Autodesk Inventor part; units mm, degrees
ref_plane "YZ Plane" through (0, 0, 0) normal (1, 0, 0) x (0, 1, 0)
ref_plane "XZ Plane" through (0, 0, 0) normal (0, 1, 0) x (-1, 0, 0)
ref_plane "XY Plane" through (0, 0, 0) normal (0, 0, 1) x (1, 0, 0)
sketch "Sketch1" plane through (0, 0, 0) normal (1, 0, 0) x (0, 1, 0)
  circle A0 centre (0, 0) radius 26.5
  dimension "d0" = 53
extrude "Extrusion1" add sketch "Sketch1" along normal blind 51
sketch "Sketch2" plane through (0, 0, 0) normal (0, 1, 0) x (-1, 0, 0)
  line L0 (-51, 26.5) -> (-51, -26.5)
  circle A0 centre (-51, 0) radius 46
  point P0 (0, 0)
  dimension "d3" = 92
extrude "Extrusion2" add sketch "Sketch2" along normal mid plane 60
move or copy body "Move Body1" bodies to move or copy 1 copy no translate (15, 0, 0)
properties part number "hip"
Model file for the job. Use its own axes, mm. A direction names the side the tool comes from. Give positions to 0.01 mm unless a question says otherwise; leave off trailing zeros. Loops run counter-clockwise (first coordinate to the right, second up) from the corner with the lowest first, then second, coordinate; pieces in that order, holes last. Notation, with made-up numbers: (-18, -8) -> (30, -8) arc R22 ccw to (30, 24) -> close; hole circle Ø3 at (16.5, 1). An arc over 180 degrees is marked (long way). Write each question's results on one line, items separated by ' | '.
(1) Cut at A-A on z = 14. List the corners of the cut face in (x, y), and give its area (3 significant figures).
Geometry results:
outline: (15, -22.5) -> (22.18, -22.5) -> (22.18, -30) -> (109.82, -30) -> (109.82, 30) -> (22.18, 30) -> (22.18, 22.5) -> (15, 22.5) -> close | area: 5,580 mm²
(2) Probe line 1 along Z through (x, y) = (69.5, 17); line 2 along X through (y, z) = (24, 32.5); line 3 along X through (y, z) = (3.5, 30.5). List the from-to ranges inside material, lowest first.
Geometry results:
line 1: z = -45.87 to 45.87 | line 2: x = 33.45 to 98.55 | line 3: x = 31.57 to 100.43
(3) Flat gauge pin, fed straight in: pin 1 Ø4 at (x, y) = (73, 17) entering from -Z. Where does the tip first touch, or does it go through?
Geometry results:
pin 1: stops at z = -45.73
(4) Cut at B-B on y = 0. List the corners of the cut face in (x, z).
Geometry results:
outline: (15, -26.5) -> (28.4, -26.5) arc R46 ccw (long way) to (28.4, 26.5) -> (15, 26.5) -> close
(5) Cut at C-C on x = 79.5. List the corners of the cut face in (y, z), and give its area (3 significant figures).
Geometry results:
outline: (-30, -43.97) -> (30, -43.97) -> (30, 43.97) -> (-30, 43.97) -> close | area: 5,280 mm²
(6) Tool access for faces 1 (the cylindrical face through (20.1, 24.5, 10.1)), 2 (the flat face through (67, -30, 1)): list every direction of +Z, -Z, +X, -X, +Y, -Y with a clear straight run to the whole face (end or side of a thin tool).
Geometry results:
face 1: -X | face 2: +Z, -Z, +X, -X, -Y
